from build123d import *

# Parameters (mm, degrees)
ESBO_O1_W                                   = 118
ESBO_O1_H                                   = 62
RESSALTO_EXTRUS_O1_DEPTH                    = 30
CORTE_EXTRUS_O1_DEPTH                       = 20
RESSALTO_EXTRUS_O2_START                    = 8
RESSALTO_EXTRUS_O2_DEPTH                    = 8
ESBO_O4_R                                   = 9
ESBO_O4_R_2                                 = 13
CORTE_EXTRUS_O2_DEPTH                       = 8
ESBO_O5_R                                   = 2
CORTE_EXTRUS_O3_DEPTH                       = 8
CORTE_EXTRUS_O4_DEPTH                       = 4
BROCA_DE_ROSQUEAR_PARA_TARRAXA_DE_M52_D     = 4.2
BROCA_DE_ROSQUEAR_PARA_TARRAXA_DE_M52_DEPTH = 13
BROCA_DE_ROSQUEAR_PARA_TARRAXA_DE_M52_TIP   = 1.2618073
FURO_COM_FOLGA_DE_M41_D                     = 4.5
ESBO_O17_W                                  = 118
ESBO_O17_H                                  = 62
ESBO_O17_W_2                                = 112.82
ESBO_O17_H_2                                = 57
CORTE_EXTRUS_O5_DEPTH                       = 77.560841819
BROCA_DE_ROSQUEAR_PARA_TARRAXA_DE_M54_D     = 4.2
BROCA_DE_ROSQUEAR_PARA_TARRAXA_DE_M54_DEPTH = 15
BROCA_DE_ROSQUEAR_PARA_TARRAXA_DE_M54_TIP   = 1.2618073
BROCA_DE_ROSQUEAR_PARA_TARRAXA_DE_M55_D     = 4.2
BROCA_DE_ROSQUEAR_PARA_TARRAXA_DE_M55_DEPTH = 15
BROCA_DE_ROSQUEAR_PARA_TARRAXA_DE_M55_TIP   = 1.2618073
ESBO_O25_R                                  = 9
CORTE_EXTRUS_O6_DEPTH                       = 69.29211155
BROCA_DE_ROSQUEAR_PARA_TARRAXA_DE_M56_D     = 4.2
BROCA_DE_ROSQUEAR_PARA_TARRAXA_DE_M56_DEPTH = 8
BROCA_DE_ROSQUEAR_PARA_TARRAXA_DE_M56_TIP   = 1.2618073
FURO_COM_FOLGA_DE_M51_D                     = 5.5
ESBO_O30_R                                  = 7.25
CORTE_EXTRUS_O9_DEPTH                       = 10


with BuildPart() as part:
    # Esboço1 → Ressalto-extrusão1 (new body)
    with BuildSketch(Plane.XY):
        with Locations((4.25, 0)):
            Rectangle(ESBO_O1_W, ESBO_O1_H)
    extrude(amount=RESSALTO_EXTRUS_O1_DEPTH)

    # Esboço2 → Corte-extrusão1 (cut)
    with BuildSketch(Plane.XY.offset(30)):
        with BuildLine():
            Line((-23.75, 26), (32.25, 26))
            ThreePointArc((32.25, 26), (58.25, 0), (32.25, -26))
            Line((32.25, -26), (-23.75, -26))
            ThreePointArc((-23.75, -26), (-49.75, 0), (-23.75, 26))
        make_face()
    extrude(amount=-CORTE_EXTRUS_O1_DEPTH, mode=Mode.SUBTRACT)

    # Esboço3 → Ressalto-extrusão2 (add)
    with BuildSketch(Plane.XY.offset(10).offset(RESSALTO_EXTRUS_O2_START)):
        with BuildLine():
            Line((51, 18.012148678), (51, -18.012148678))
            ThreePointArc((51, -18.012148678), (58.25, 0), (51, 18.012148678))
        make_face()
    extrude(amount=-RESSALTO_EXTRUS_O2_DEPTH)

    # Esboço4 → Corte-extrusão2 (cut)
    with BuildSketch(Plane.XY.offset(10)):
        with Locations((-30.5, 0)):
            Circle(ESBO_O4_R)
        Circle(ESBO_O4_R_2)
        with Locations((33, 0)):
            Circle(ESBO_O4_R_2)
    extrude(amount=-CORTE_EXTRUS_O2_DEPTH, mode=Mode.SUBTRACT)

    # Esboço5 → Corte-extrusão3 (cut)
    with BuildSketch(Plane.XY.offset(30)):
        with Locations((-47.25, 18)):
            Circle(ESBO_O5_R)
        with Locations((55.75, 18)):
            Circle(ESBO_O5_R)
        with Locations((55.75, -18)):
            Circle(ESBO_O5_R)
        with Locations((-47.25, -18)):
            Circle(ESBO_O5_R)
    extrude(amount=-CORTE_EXTRUS_O3_DEPTH, mode=Mode.SUBTRACT)

    # Esboço6 → Corte-extrusão4 (cut)
    with BuildSketch(Plane.XY.offset(10)):
        with BuildLine():
            Line((-38.985281374, 3), (-43.985281374, 3))
            ThreePointArc((-43.985281374, 3), (-46.985281374, 0), (-43.985281374, -3))
            Line((-43.985281374, -3), (-38.985281374, -3))
            Line((-38.985281374, -3), (-38.985281374, 3))
        make_face()
        with BuildLine():
            Line((-33.5, 8.485281374), (-27.5, 8.485281374))
            Line((-27.5, 8.485281374), (-27.5, 13.485281374))
            ThreePointArc((-27.5, 13.485281374), (-30.5, 16.485281374), (-33.5, 13.485281374))
            Line((-33.5, 13.485281374), (-33.5, 8.485281374))
        make_face()
        with BuildLine():
            Line((-33.5, -8.485281374), (-33.5, -13.485281374))
            ThreePointArc((-33.5, -13.485281374), (-30.5, -16.485281374), (-27.5, -13.485281374))
            Line((-27.5, -13.485281374), (-27.5, -8.485281374))
            Line((-27.5, -8.485281374), (-33.5, -8.485281374))
        make_face()
    extrude(amount=-CORTE_EXTRUS_O4_DEPTH, mode=Mode.SUBTRACT)

    # Broca de rosquear para tarraxa de M52
    with Locations(Plane.XY.offset(30)):
        with Locations((-44.07, 23), (-44.07, -23), (52.25, -23), (52.25, 23)):
            Hole(BROCA_DE_ROSQUEAR_PARA_TARRAXA_DE_M52_D / 2, depth=BROCA_DE_ROSQUEAR_PARA_TARRAXA_DE_M52_DEPTH)
            with Locations((0, 0, -(BROCA_DE_ROSQUEAR_PARA_TARRAXA_DE_M52_DEPTH + BROCA_DE_ROSQUEAR_PARA_TARRAXA_DE_M52_TIP / 2))):  # 118° drill point
                Cone(0, BROCA_DE_ROSQUEAR_PARA_TARRAXA_DE_M52_D / 2, BROCA_DE_ROSQUEAR_PARA_TARRAXA_DE_M52_TIP, mode=Mode.SUBTRACT)

    # Furo com folga de M41 (through all)
    with Locations(Plane.XY.offset(6)):
        with Locations((-30.5, -12.5), (-43, 0), (-30.5, 12.5)):
            Hole(FURO_COM_FOLGA_DE_M41_D / 2)

    # Esboço17 → Corte-extrusão5 (cut, through all)
    with BuildSketch(Plane.XY.offset(30)):
        with Locations((4.25, 0)):
            Rectangle(ESBO_O17_W, ESBO_O17_H)
        with Locations((2.34, 0)):
            Rectangle(ESBO_O17_W_2, ESBO_O17_H_2, mode=Mode.SUBTRACT)
    extrude(amount=-CORTE_EXTRUS_O5_DEPTH, mode=Mode.SUBTRACT)

    # Broca de rosquear para tarraxa de M54
    with Locations(Plane(origin=(0, -28.5, 0), x_dir=(-1, 0, 0), z_dir=(0, -1, 0))):
        with Locations((-51.75, -4), (-16.25, -4)):
            Hole(BROCA_DE_ROSQUEAR_PARA_TARRAXA_DE_M54_D / 2, depth=BROCA_DE_ROSQUEAR_PARA_TARRAXA_DE_M54_DEPTH)
            with Locations((0, 0, -(BROCA_DE_ROSQUEAR_PARA_TARRAXA_DE_M54_DEPTH + BROCA_DE_ROSQUEAR_PARA_TARRAXA_DE_M54_TIP / 2))):  # 118° drill point
                Cone(0, BROCA_DE_ROSQUEAR_PARA_TARRAXA_DE_M54_D / 2, BROCA_DE_ROSQUEAR_PARA_TARRAXA_DE_M54_TIP, mode=Mode.SUBTRACT)

    # Broca de rosquear para tarraxa de M55
    with Locations(Plane(origin=(0, 28.5, 0), x_dir=(1, 0, 0), z_dir=(0, 1, 0))):
        with Locations((51.75, -4), (16.25, -4)):
            Hole(BROCA_DE_ROSQUEAR_PARA_TARRAXA_DE_M55_D / 2, depth=BROCA_DE_ROSQUEAR_PARA_TARRAXA_DE_M55_DEPTH)
            with Locations((0, 0, -(BROCA_DE_ROSQUEAR_PARA_TARRAXA_DE_M55_DEPTH + BROCA_DE_ROSQUEAR_PARA_TARRAXA_DE_M55_TIP / 2))):  # 118° drill point
                Cone(0, BROCA_DE_ROSQUEAR_PARA_TARRAXA_DE_M55_D / 2, BROCA_DE_ROSQUEAR_PARA_TARRAXA_DE_M55_TIP, mode=Mode.SUBTRACT)

    # Esboço25 → Corte-extrusão6 (cut, through all)
    with BuildSketch(Plane.XY.offset(10)):
        with Locations((-30.5, 0)):
            Circle(ESBO_O25_R)
    extrude(amount=-CORTE_EXTRUS_O6_DEPTH, mode=Mode.SUBTRACT)

    # Broca de rosquear para tarraxa de M56
    with Locations(Plane(origin=(0, 0, 0), x_dir=(-1, 0, 0), z_dir=(0, 0, -1))):
        with Locations((47.123, 21.276), (47.123, -21.276), (13.877, -21.28), (13.877, 21.28)):
            Hole(BROCA_DE_ROSQUEAR_PARA_TARRAXA_DE_M56_D / 2, depth=BROCA_DE_ROSQUEAR_PARA_TARRAXA_DE_M56_DEPTH)
            with Locations((0, 0, -(BROCA_DE_ROSQUEAR_PARA_TARRAXA_DE_M56_DEPTH + BROCA_DE_ROSQUEAR_PARA_TARRAXA_DE_M56_TIP / 2))):  # 118° drill point
                Cone(0, BROCA_DE_ROSQUEAR_PARA_TARRAXA_DE_M56_D / 2, BROCA_DE_ROSQUEAR_PARA_TARRAXA_DE_M56_TIP, mode=Mode.SUBTRACT)

    # Furo com folga de M51 (through all)
    with Locations(Plane.XY.offset(2)):
        with Locations((33, 0)):
            Hole(FURO_COM_FOLGA_DE_M51_D / 2)

    # Esboço30 → Corte-extrusão9 (cut)
    with BuildSketch(Plane.XY.offset(2)):
        Circle(ESBO_O30_R)
    extrude(amount=-CORTE_EXTRUS_O9_DEPTH, mode=Mode.SUBTRACT)


solid = part.part
Read the model definition and answer for the solid it produces. Units are mm, in the model's axes. A direction names the side the tool comes from. Give positions to 0.01 mm unless a question says otherwise; leave off trailing zeros. Loops run counter-clockwise (first coordinate to the right, second up) from the corner with the lowest first, then second, coordinate; pieces in that order, holes last. Notation, with made-up numbers: (83, -2) -> (112, -2) arc R9 cw to (112, 9) -> close; hole circle Ø8 at (-15, 13.5). An arc over 180 degrees is marked (long way). Answer as CSV lines item,"result".
Item 1: For faces 4 (the face through (51.12, 24.77, 23.41)), 5 (the face through (15.886, 12.457, 3.984)), determine the directions among +Z, -Z, +X, -X, +Y, -Y from which every point of the face is accessible in a straight line to the end or side of a thin tool.
Returned:
face 4,"+Z"
face 5,"+Y"
Item 2: Find section A-A on z = 13.5. Give the vertices of the cut face in (x, y), plus the area to 3 significant figures.
Returned:
outline,"(-54.07, -28.5) -> (58.75, -28.5) -> (58.75, 28.5) -> (-54.07, 28.5) -> close; hole (-23.75, -26) -> (32.25, -26) arc R26 ccw to (51, -18.01) -> (51, 18.01) arc R26 ccw to (32.25, 26) -> (-23.75, 26) arc R26 ccw to start"
area,"1,570 mm²"
Item 3: Consider line 1 (Z direction, x = 16, y = 21); line 2 (Y direction, x = 18, z = 16); line 3 (Y direction, x = 0, z = 8). Determine where each line is inside the solid, lowest interval first. Write a range as [from, to].
Returned:
line 1,"z = [0, 1.91], [6.09, 10]"
line 2,"y = [-28.5, -26], [26, 28.5]"
line 3,"y = [-28.5, -13], [13, 28.5]"
Item 4: Determine the mould class of faces 1 (the face through (58.75, 0, 15)), 2 (the face through (4, 26, 20)), 3 (the face through (2, 28.5, 15)) for opening direction X: +X half, -X half, draft (parallel to the pull), parting line (faces both ways), or undercut.
Returned:
face 1,"+X half"
face 2,"undercut"
face 3,"draft"
Item 5: Find section B-B on z = 24. State how many separate pieces and enclosed holes the cut face has, plus the area to 3 significant figures.
Returned:
separate pieces,"1"
enclosed holes,"9"
area,"1,290 mm²"
Item 6: Each of these flat-tipped pins is pushed along its axis until it touches: pin 1 (1.8 mm diameter, centred on x = -29.5, y = 11.5, fed in from +Z); pin 2 (3 mm diameter, centred on x = -47.25, y = 18, fed in from +Z); pin 3 (5.5 mm diameter, centred on x = -13.877, y = -21.28, fed in from +Z); pin 4 (5.5 mm diameter, centred on x = -47.123, y = 21.276, fed in from -Z). Where does it stop, or does it pass through?
Returned:
pin 1,"stops at z = 6"
pin 2,"stops at z = 22"
pin 3,"stops at z = 10"
pin 4,"stops at z = 0"
Item 7: Find section C-C on x = 42. Give the vertices of the cut face in (y, z), plus the area to 3 significant figures.
Returned:
outline,"(-28.5, 0) -> (28.5, 0) -> (28.5, 30) -> (24.1, 30) -> (24.1, 10) -> (9.38, 10) -> (9.38, 2) -> (-9.38, 2) -> (-9.38, 10) -> (-24.1, 10) -> (-24.1, 30) -> (-28.5, 30) -> close"
area,"596 mm²"
